```python
from build123d import *

# Parameters (mm, degrees)
F0_W     = 50.8
F0_H     = 50.8
F1_DEPTH = 25.4


with BuildPart() as f1:
    # F0 (on Top) → F1 (new body)
    with BuildSketch(Plane.XY):
        with Locations((-13.693494, 6.764759)):
            Rectangle(F0_W, F0_H)
        with BuildLine():
            ThreePointArc((-29.822317, 5.883413), (-28.154331, 20.718998), (-13.693494, 17.00942))
            ThreePointArc((-13.693494, 17.00942), (-2.571968, 22.202675), (5.04269, 12.575878))
            ThreePointArc((5.04269, 12.575878), (4.367831, 8.984659), (2.435328, 5.883413))
            Line((2.435328, 5.883413), (-13.693494, -11.674106))
            Line((-13.693494, -11.674106), (-29.822317, 5.883413))
        make_face(mode=Mode.SUBTRACT)
    extrude(amount=F1_DEPTH)


solid = f1.part
```
For this review, take the finished solid that the model builds, in its own axes (mm). Give positions to 0.01 mm unless a question says otherwise; leave off trailing zeros. Order: outer loops, then holes, each group sorted by start corner. A loop starts at its lowest first (then second) coordinate and runs counter-clockwise, first axis right, second up.
1) Take a section at C-C (y = 19). Give the boundary of the cut face in (x, z), then the cut area to 3 significant figures.
2) Take a section at D-D (z = 9). Give the boundary of the cut face in (x, y), then the cut area to 3 significant figures.
3) Take a section at A-A (y = 0). Give the boundary of the cut face in (x, z), then the cut area to 3 significant figures.
4) The part is to be moulded in two halves that separate along Y. For faces 1 (the face through (-14, 18, 0)), 2 (the face through (-14, -18.635, 13)), 3 (the face through (-5.516, -2.772, 12.522)), 4 (the face through (-21.645, -3.018, 12.522)), say which applies: released by +Y, released by -Y, zero draft, split by the parting line, or undercut.
5) Take a section at B-B (x = -3). Give the boundary of the cut face in (y, z).
6) Wall thickness on line 1 (X direction, y = 18, z = 3.25); line 2 (X direction, y = 9, z = 17.75); line 3 (Y direction, x = -18.5, z = 13.75): over which ranges is each line inside the solid? List them lowest first.
Derived:
1. outline: (-39.09, 0) - (-30.06, 0) - (-30.06, 25.4) - (-39.09, 25.4) - close; (-15.01, 0) - (-12.37, 0) - (-12.37, 25.4) - (-15.01, 25.4) - close; (2.67, 0) - (11.71, 0) - (11.71, 25.4) - (2.67, 25.4) - close
1. area: 526 mm2
2. outline: (-39.09, -18.64) - (11.71, -18.64) - (11.71, 32.16) - (-39.09, 32.16) - close; hole (-29.82, 5.88) - (-13.69, -11.67) - (2.44, 5.88) arc R9.89 ccw to (5.04, 12.58) arc R9.89 ccw to (-13.69, 17.01) arc R9.89 ccw (long way) to start
2. area: 1,760 mm2
3. outline: (-39.09, 0) - (-24.42, 0) - (-24.42, 25.4) - (-39.09, 25.4) - close; (-2.97, 0) - (11.71, 0) - (11.71, 25.4) - (-2.97, 25.4) - close
3. area: 746 mm2
4. face 1: zero draft
4. face 2: released by -Y
4. face 3: undercut
4. face 4: undercut
5. outline: (-18.64, 0) - (-0.03, 0) - (-0.03, 25.4) - (-18.64, 25.4) - close; (22.29, 0) - (32.16, 0) - (32.16, 25.4) - (22.29, 25.4) - close
6. line 1: x = -39.09 to -30.81, -14.26 to -13.12, 3.42 to 11.71
6. line 2: x = -39.09 to -31.76, 4.37 to 11.71
6. line 3: y = -18.64 to -6.44, 21.61 to 32.16
